Check sheet for the modelled part. Datum: model origin and axes. Units: mm. A direction names the side the tool comes from. Round coordinates to 2 decimals unless told otherwise and drop trailing zeros. Loops run counter-clockwise (first coordinate to the right, second up) from the corner with the lowest first, then second, coordinate; pieces in that order, holes last. Notation, with made-up numbers: (33, 79.25) -> (49, 79.25) arc R16 ccw to (49, 84.25) -> close; hole circle Ø3 at (44.5, 60.5). An arc over 180 degrees is marked (long way). Use one line per item in the form item = value. Start each with the question number.
(1) Set-up check for faces 4 (the cylindrical face through (0, 10, 3)), 5 (the cylindrical face through (-0.1, 5.5, 6.2)): record each of +Z, -Z, +X, -X, +Y, -Y from which the full face is reachable in a straight line by a thin tool's end or side.
(2) Sectioned sample at C-C (y = 8). Record the cut outline in (x, z), and give its area (3 significant figures).
(3) Sectioned sample at D-D (y = -5). Record the cut outline in (x, z), and give its area (3 significant figures).
(4) Go/stop test with flat-tipped pins: pin 1 (2 mm diameter, centred on x = -3.5, z = 2.5, fed in from -Y); pin 2 (3 mm diameter, centred on y = -11, z = 3, fed in from -X); pin 3 (5 mm diameter, centred on x = -6.5, y = -5, fed in from +Z). Record where each tip stops, or that it passes through.
(5) Sectioned sample at B-B (z = 3). Record the cut outline in (x, y), and give its area (3 significant figures).
(6) Sectioned sample at A-A (x = 0). Record the cut outline in (y, z).
(7) Material ranges on probe 1 along Z at (x, y) = (0, -12); probe 2 along Z at (x, y) = (-9, -6); probe 3 along X at (y, z) = (8.5, 4.25), recorded low to high. Write a range as [from, to].
(8) Draft check along X on faces 1 (the cylindrical face through (-1.31, -9.24, 4)), 2 (the flat face through (0, -7, 6)), 3 (the cylindrical face through (0.1, -5.5, 6.2)). Enter one of: released by +X, released by -X, zero draft, split by the parting line, or undercut.
from build123d import *

# Parameters (mm, degrees)
SKETCH_1_R            = 4
SKETCH_1_R_2          = 2
EXTRUDE_1_DEPTH       = 6
SKETCH_2_R            = 4
EXTRUDE_2_DEPTH       = 0.5
SKETCH_5_R            = 2.747111961
EXTRUDE_3_DEPTH       = 6.5
HOLE_WIZARD_M41_D     = 3.3
HOLE_WIZARD_M41_DEPTH = 16.499
HOLE_WIZARD_M41_TIP   = 0.991420021
CUT_EXTRUDE_1_DEPTH   = 6.5


with BuildPart() as part:
    # Эскиз1 → Бобышка-Вытянуть1 (new body)
    with BuildSketch(Plane.XY):
        with BuildLine():
            Line((-5.5, 0), (-3.937070517, 8.70673598))
            ThreePointArc((-3.937070517, 8.70673598), (0, 12), (3.937070517, 8.70673598))
            Line((3.937070517, 8.70673598), (5.5, 0))
            Line((5.5, 0), (14.456832295, -4))
            ThreePointArc((14.456832295, -4), (0, -15), (-14.456832295, -4))
            Line((-14.456832295, -4), (-5.5, 0))
        make_face()
        Circle(SKETCH_1_R, mode=Mode.SUBTRACT)
        with Locations((0, 8)):
            Circle(SKETCH_1_R_2, mode=Mode.SUBTRACT)
    extrude(amount=EXTRUDE_1_DEPTH)

    # Эскиз2 → Бобышка-Вытянуть2 (add)
    with BuildSketch(Plane.XY.offset(6)):
        with BuildLine():
            Line((5.156610425, 1.912947706), (5.5, 0))
            ThreePointArc((5.5, 0), (0, -5.5), (-5.5, 0))
            Line((-5.5, 0), (-5.156610425, 1.912947706))
            ThreePointArc((-5.156610425, 1.912947706), (0, 5.5), (5.156610425, 1.912947706))
        make_face()
        Circle(SKETCH_2_R, mode=Mode.SUBTRACT)
    extrude(amount=EXTRUDE_2_DEPTH)

    # Эскиз5 → Бобышка-Вытянуть3 (add)
    with BuildSketch(Plane(origin=(0, -10, 0), x_dir=(1, 0, 0), z_dir=(0, 1, 0))):
        with Locations((0, -3)):
            Circle(SKETCH_5_R)
    extrude(amount=-EXTRUDE_3_DEPTH)

    # Отверстие обработанное метчиком M41
    with Locations(Plane(origin=(0, -16.5, 0), x_dir=(-1, 0, 0), z_dir=(0, -1, 0))):
        with Locations((0, -3)):
            Hole(HOLE_WIZARD_M41_D / 2, depth=HOLE_WIZARD_M41_DEPTH)
            with Locations((0, 0, -(HOLE_WIZARD_M41_DEPTH + HOLE_WIZARD_M41_TIP / 2))):  # 118° drill point
                Cone(0, HOLE_WIZARD_M41_D / 2, HOLE_WIZARD_M41_TIP, mode=Mode.SUBTRACT)

    # Эскиз8 → Вырез-Вытянуть1 (cut)
    with BuildSketch(Plane.XY.offset(6)):
        with BuildLine():
            Line((-5.46363589, -13.96956273), (-5.46363589, -17.421493936))
            ThreePointArc((-5.46363589, -17.421493936), (0, -18.258142515), (5.46363589, -17.421493936))
            Line((5.46363589, -17.421493936), (5.46363589, -13.96956273))
            ThreePointArc((5.46363589, -13.96956273), (0, -15), (-5.46363589, -13.96956273))
        make_face()
    extrude(amount=-CUT_EXTRUDE_1_DEPTH, mode=Mode.SUBTRACT)


solid = part.part
Checks:
q1.face_4 = +Z, -Z
q1.face_5 = +Z, +Y
q2.outline = (-4.06, 0) -> (-2, 0) -> (-2, 6) -> (-4.06, 6) -> close; (2, 0) -> (4.06, 0) -> (4.06, 6) -> (2, 6) -> close
q2.area = 24.8 mm2
q3.outline = (-14.14, 0) -> (14.14, 0) -> (14.14, 6) -> (2.29, 6) -> (2.29, 6.5) -> (-2.29, 6.5) -> (-2.29, 6) -> (-14.14, 6) -> close; hole circle Ø3.3 at (0, 3)
q3.area = 163 mm2
q4.pin_1 = -14.79
q4.pin_2 = -11.61
q4.pin_3 = 6
q5.outline = (-14.46, -4) arc R15 ccw to (-1.65, -14.91) -> (-1.65, -3.64) arc R4 cw (long way) to (1.65, -3.64) -> (1.65, -14.91) arc R15 ccw to (14.46, -4) -> (5.5, 0) -> (3.94, 8.71) arc R4 ccw to (-3.94, 8.71) -> (-5.5, 0) -> close; hole circle Ø4 at (0, 8)
q5.area = 317 mm2
q6.outline = (-15, 0) -> (-4, 0) -> (-4, 1.35) -> (-15, 1.35) -> close; (-15, 4.65) -> (-4, 4.65) -> (-4, 6.5) -> (-5.5, 6.5) -> (-5.5, 6) -> (-15, 6) -> close; (4, 0) -> (6, 0) -> (6, 6) -> (5.5, 6) -> (5.5, 6.5) -> (4, 6.5) -> close; (10, 0) -> (12, 0) -> (12, 6) -> (10, 6) -> close
q7.probe_1 = [0, 1.35], [4.65, 6]
q7.probe_2 = [0, 6]
q7.probe_3 = [-3.97, -1.94], [1.94, 3.97]
q8.face_1 = undercut
q8.face_2 = zero draft
q8.face_3 = split by the parting line
